```python
from build123d import *

# Parameters (mm, degrees)
SKETCH1_W               = 14
SKETCH1_H               = 3.5
BOSS_EXTRUDE1_DEPTH     = 1.9
BOSS_EXTRUDE2_DEPTH     = 0.4
CUT_EXTRUDE1_DEPTH      = 50.105702317
CUT_EXTRUDE1_DEPTH_BACK = 50.105702317
SKETCH4_W               = 0.07
SKETCH4_H               = 0.024
BOSS_EXTRUDE3_DEPTH     = 10


with BuildPart() as part:
    # Sketch1 → Boss-Extrude1 (new body)
    with BuildSketch(Plane(origin=(0, 0, 0), x_dir=(1, 0, 0), z_dir=(0, 1, 0))):
        Rectangle(SKETCH1_W, SKETCH1_H)
    extrude(amount=BOSS_EXTRUDE1_DEPTH)

    # Sketch2 → Boss-Extrude2 (add)
    with BuildSketch(Plane.XZ):
        Polygon((7, -1.75), (7.5, -1.75), (8.35, -2.6), (49, -2.6), (49, 2.6), (8.35, 2.6), (7.5, 1.75), (7, 1.75), align=None)
        with BuildLine():
            Line((47.175, 1.1), (10.175, 1.1))
            ThreePointArc((10.175, 1.1), (9.675, 1.6), (10.175, 2.1))
            Line((10.175, 2.1), (47.175, 2.1))
            ThreePointArc((47.175, 2.1), (47.675, 1.6), (47.175, 1.1))
        make_face(mode=Mode.SUBTRACT)
        with BuildLine():
            Line((47.175, -2.1), (10.175, -2.1))
            ThreePointArc((10.175, -2.1), (9.675, -1.6), (10.175, -1.1))
            Line((10.175, -1.1), (47.175, -1.1))
            ThreePointArc((47.175, -1.1), (47.675, -1.6), (47.175, -2.1))
        make_face(mode=Mode.SUBTRACT)
    extrude(amount=-BOSS_EXTRUDE2_DEPTH)

    # Sketch3 → Cut-Extrude1 (cut, two sides: drawn at the far end of the back side and taken through both)
    with BuildSketch(Plane.XY.offset(-CUT_EXTRUDE1_DEPTH_BACK)):
        with BuildLine():
            Line((7, 0.6), (7, 1.9))
            Line((7, 1.9), (2, 1.9))
            ThreePointArc((2, 1.9), (3.291559135, 1.734842828), (4.5, 1.25))
            ThreePointArc((4.5, 1.25), (5.708440865, 0.765157172), (7, 0.6))
        make_face()
    extrude(amount=CUT_EXTRUDE1_DEPTH + CUT_EXTRUDE1_DEPTH_BACK, mode=Mode.SUBTRACT)

    # Sketch4 → Boss-Extrude3 (add)
    with BuildSketch(Plane.ZY.offset(7)):
        with Locations((0, 0.5)):
            Rectangle(SKETCH4_W, SKETCH4_H)
    extrude(amount=BOSS_EXTRUDE3_DEPTH)


solid = part.part
```
Work out the finished part from the listing and answer in its coordinate system (mm). A direction names the side the tool comes from. Coordinates: 2 decimals unless noted, no trailing zeros. Order: outer loops, then holes, each group sorted by start corner. A loop starts at its lowest first (then second) coordinate and runs counter-clockwise, first axis right, second up. Notation, with made-up numbers: M 10,59.25 L 62,59.25 A23 ccw 62,98.25 Z; hole C 13.25,-8 d7. An arc over 180 degrees is marked long. Use CSV: the item, a comma, the result in double quotes.
1) For faces 1 (the face through (28, 0.4, 0)), 2 (the face through (-3, 1.9, 0)), determine the directions among +Z, -Z, +X, -X, +Y, -Y from which every point of the face is accessible in a straight line to the end or side of a thin tool.
Worked out:
face 1,"+Z, -Z, +X, +Y"
face 2,"+Z, -Z, +X, -X, +Y"
2) Determine the mould class of faces 3 (the face through (-1, 1, -1.75)), 4 (the face through (21, 0, 0)), 5 (the face through (-1, 1, 1.75)) for opening direction Z: released by +Z, released by -Z, zero draft, split by the parting line, or undercut.
Worked out:
face 3,"released by -Z"
face 4,"zero draft"
face 5,"released by +Z"
3) Consider line 1 (Z direction, x = 39.5, y = 0.25); line 2 (X direction, y = 0.25, z = 0.8); line 3 (Y direction, x = 15, z = 0.5). Determine where each line is inside the solid, lowest interval first. Write a range as [from, to].
Worked out:
line 1,"z = [-2.6, -2.1], [-1.1, 1.1], [2.1, 2.6]"
line 2,"x = [-7, 49]"
line 3,"y = [0, 0.4]"
4) Flat-ended cylindrical pins translate along their axes: pin 1 Ø1 at (y, z) = (1, -1) entering from -X; pin 2 Ø0.6 at (x, y) = (-1, 1) entering from +Z; pin 3 Ø0.6 at (x, y) = (1, 1) entering from -Z. Find the tip coordinate at first contact, or state that the pin passes through.
Worked out:
pin 1,"stops at x = -7"
pin 2,"stops at z = 1.75"
pin 3,"stops at z = -1.75"
5) Section A-A on x = 28.5 is taken. Write down the section's boundary in (y, z).
Worked out:
outline,"M 0,-2.6 L 0.4,-2.6 L 0.4,-2.1 L 0,-2.1 Z; M 0,-1.1 L 0.4,-1.1 L 0.4,1.1 L 0,1.1 Z; M 0,2.1 L 0.4,2.1 L 0.4,2.6 L 0,2.6 Z"
